Design review of the part shown in the three views and the two pictorial views. Dimensions are in mm from the part's minimum x, y and z. A direction names the side the tool comes from. Give positions to 0.01 mm unless a question says otherwise; leave off trailing zeros. Loops run counter-clockwise (first coordinate to the right, second up) from the corner with the lowest first, then second, coordinate; pieces in that order, holes last. Notation, with made-up numbers: (3.5, 60.25) -> (30.5, 60.25) arc R32 cw to (30.5, 90.25) -> close; hole circle Ø2 at (43, 86). An arc over 180 degrees is marked (long way). Use CSV: the item, a comma, the result in double quotes. Start each with the question number.
Item 1: We need section A-A (y = 30). State the section outline as (x, z) points.
Item 2: We need section B-B (x = 30). State the section outline as (y, z) points, plus the area to 3 significant figures.
Item 3: We need section D-D (z = 8). Count the separate pieces of the cut face and the enclosed holes in it, plus the area to 3 significant figures.
Item 4: For the marked faces 1 and 2, list the 3-axis set-ups (+Z, -Z, +X, -X, +Y, -Y) from which the entire face can be reached by the end or side of a thin tool; tool diameter is ignored.
Item 5: Wall thickness on line 1 along Y through (x, z) = (30, 7.85); line 2 along Y through (x, z) = (13.5, 8.5) (1 decimal); line 3 along X through (y, z) = (7, 8.25) (1 decimal): over which ranges is each line inside the solid? List them lowest first. Write a range as from..to.
Item 6: The part is to be moulded in two halves that separate along X. For the marked faces 3, 4 and 5, say which applies: +X half, -X half, draft (parallel to the pull), parting line (faces both ways), or undercut.
Item 7: We need section C-C (y = 5). State the section outline as (x, z) points (1 decimal).
Item 8: Clearance check with flat-ended pins moving along their axes: pin 1 (6 mm diameter, centred on x = 21.45, y = 6.51, fed in from -Z); pin 2 (5 mm diameter, centred on y = 43, z = 4, fed in from +X); pin 3 (3 mm diameter, centred on y = 6.5, z = 7.5, fed in from +X) (1 decimal). State where each tip first meets the part, or that it passes through.
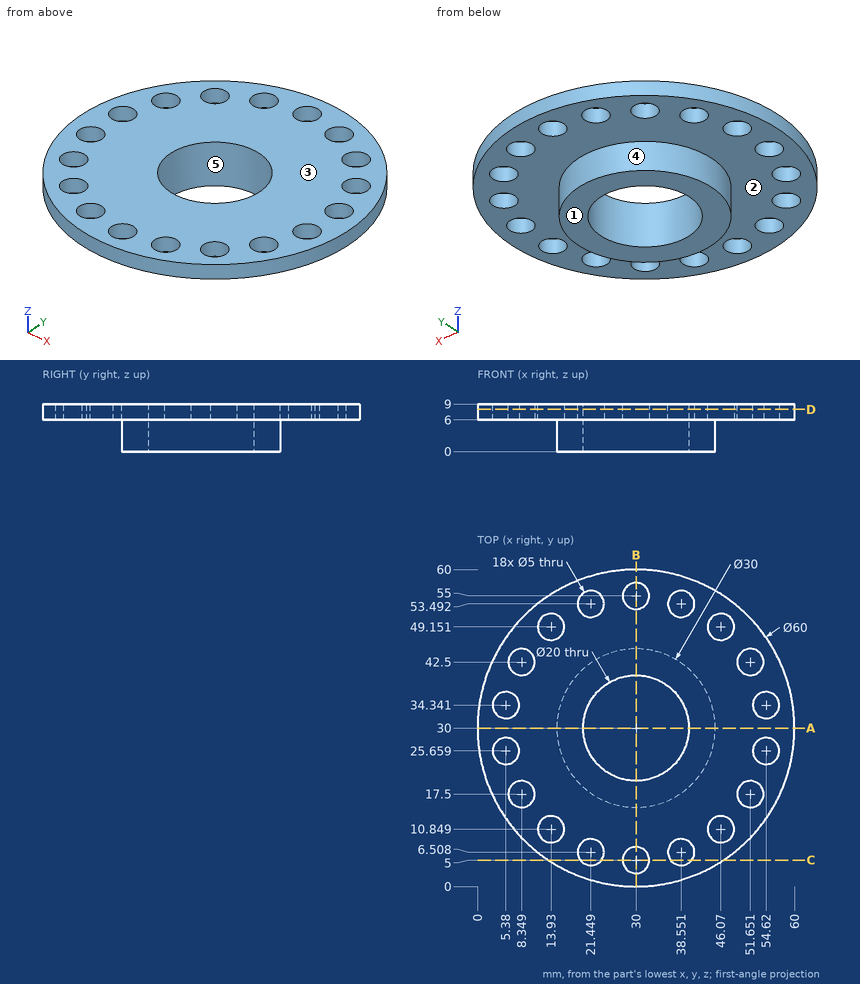
Results found:
1,outline,"(0, 6) -> (15, 6) -> (15, 0) -> (20, 0) -> (20, 9) -> (0, 9) -> close; (40, 0) -> (45, 0) -> (45, 6) -> (60, 6) -> (60, 9) -> (40, 9) -> close"
2,outline,"(0, 6) -> (2.5, 6) -> (2.5, 9) -> (0, 9) -> close; (7.5, 6) -> (15, 6) -> (15, 0) -> (20, 0) -> (20, 9) -> (7.5, 9) -> close; (40, 0) -> (45, 0) -> (45, 6) -> (52.5, 6) -> (52.5, 9) -> (40, 9) -> close; (57.5, 6) -> (60, 6) -> (60, 9) -> (57.5, 9) -> close"
2,area,"150 mm²"
3,separate pieces,"1"
3,enclosed holes,"19"
3,area,"2,160 mm²"
4,face 1,"-Z, +X, -X, +Y, -Y"
4,face 2,"-Z"
5,line 1,"0..2.5, 7.5..20, 40..52.5, 57.5..60"
5,line 2,"4.9..8.4, 13.3..46.7, 51.6..55.1"
5,line 3,"10.7..19, 23.9..28.5, 31.5..36.1, 41..49.3"
6,face 3,"draft"
6,face 4,"parting line"
6,face 5,"undercut"
7,outline,"(13.4, 6) -> (19.5, 6) -> (19.5, 9) -> (13.4, 9) -> close; (23.4, 6) -> (27.5, 6) -> (27.5, 9) -> (23.4, 9) -> close; (32.5, 6) -> (36.6, 6) -> (36.6, 9) -> (32.5, 9) -> close; (40.5, 6) -> (46.6, 6) -> (46.6, 9) -> (40.5, 9) -> close"
8,pin 1,"z = 6"
8,pin 2,"x = 57.71"
8,pin 3,"x = 50.4"
